Part model, mm, in its own coordinate system. Face numbers are marked on the shaded views. A direction names the side the tool comes from. Round coordinates to 2 decimals unless told otherwise and drop trailing zeros. Order: outer loops, then holes, each group sorted by start corner. A loop starts at its lowest first (then second) coordinate and runs counter-clockwise, first axis right, second up. Notation, with made-up numbers: M 86,75 L 123,75 A7 ccw 123,88 Z; hole C -33,-26 d8. An arc over 180 degrees is marked long. Write each question's results on one line, items separated by ' | '. Start each with the question number.
1. Band-saw the part on C-C, the plane z = 80.5. List the corners of the cut face in (x, y).
2. Probe L1, parallel to Y at x = 274, z = 66; L2, parallel to Z at x = 535, y = 53; L3, parallel to Y at x = 479.5, z = 6. List the from-to ranges inside material, lowest first. Write a range as [from, to].
3. Band-saw the part on B-B, the plane y = 52.5. List the corners of the cut face in (x, z), then the cut area to 3 significant figures.
4. Band-saw the part on D-D, the plane x = 56. List the corners of the cut face in (y, z), then the cut area to 3 significant figures.
5. Which spindle directions (+Z, -Z, +X, -X, +Y, -Y) get a long thin tool onto all of the face, cutting with end or side? Do the marked faces 1 and 2. Say none if no direction does.
6. Band-saw the part on A-A, the plane x = 571.5. List the corners of the cut face in (y, z).
7. Drop flat-ended pins along their axis: pin 1 Ø1 at (x, z) = (447.5, 37.5) entering from +Y; pin 2 Ø8 at (x, y) = (428.5, 29.5) entering from +Z; pin 3 Ø6 at (y, z) = (51, 11.5) entering from +X. Give the stop position or say it passes through.
```python
from build123d import *

# Parameters (mm, degrees)
F1_DEPTH = 800
F3_DEPTH = 100
F5_DEPTH = 100.001


with BuildPart() as f1:
    # F0 (on Right) → F1 (new body)
    with BuildSketch(Plane.YZ):
        with BuildLine():
            Line((-12.360656, 95), (-12.360656, 0))
            Line((-12.360656, 0), (82.639344, 0))
            ThreePointArc((82.639344, 0), (86.174878, 1.464466), (87.639344, 5))
            ThreePointArc((87.639344, 5), (86.174878, 8.535534), (82.639344, 10))
            Line((82.639344, 10), (2.639344, 10))
            ThreePointArc((2.639344, 10), (-0.89619, 11.464466), (-2.360656, 15))
            Line((-2.360656, 15), (-2.360656, 95))
            ThreePointArc((-2.360656, 95), (-3.825122, 98.535534), (-7.360656, 100))
            ThreePointArc((-7.360656, 100), (-10.89619, 98.535534), (-12.360656, 95))
        make_face()
    extrude(amount=F1_DEPTH)

    # F2 (on face) → F3 (cut)
    with BuildSketch(Plane(origin=(0, 0, 0), x_dir=(1, 0, 0), z_dir=(0, 0, -1))):
        Polygon((800, -82.639344), (800, 12.360656), (705, -82.639344), align=None)
        Polygon((800, -87.639344), (800, -82.639344), (705, -82.639344), (700, -87.639344), align=None)
    extrude(amount=-F3_DEPTH, mode=Mode.SUBTRACT)

    # F4 (on face) → F5 (cut, through all)
    with BuildSketch(Plane(origin=(0, 0, 0), x_dir=(1, 0, 0), z_dir=(0, 0, -1))):
        Polygon((95, -82.639344), (0, -82.639344), (0, -87.639344), (100, -87.639344), align=None)
        Polygon((95, -82.639344), (0, 12.360656), (0, -82.639344), align=None)
    extrude(amount=-F5_DEPTH, mode=Mode.SUBTRACT)


solid = f1.part
```
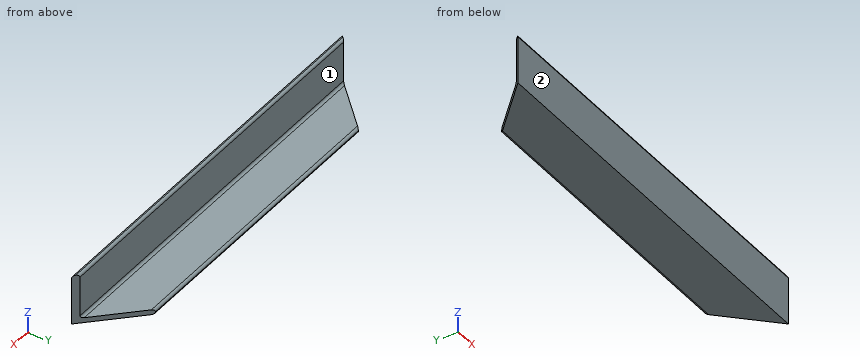
Solution:
1) outline: M 0,-12.36 L 800,-12.36 L 790,-2.36 L 10,-2.36 Z
2) L1: [-12.36, -2.36] | L2: [0, 10] | L3: [-12.36, 87.54]
3) outline: M 64.86,0 L 735.14,0 L 735.14,10 L 64.86,10 Z | area: 6,700 mm^2
4) outline: M -12.36,0 L 43.64,0 L 43.64,10 L 2.64,10 A5 cw -2.36,15 L -2.36,95 A5 ccw -12.36,95 Z | area: 1,450 mm^2
5) face 1: +Z, +X, -X, +Y | face 2: +Z, -Z, +X, -X, -Y
6) outline: M -12.36,0 L 82.64,0 A5 ccw 82.64,10 L 2.64,10 A5 cw -2.36,15 L -2.36,95 A5 ccw -12.36,95 Z
7) pin 1: y = -2.36 | pin 2: z = 10 | pin 3: x = 739.24
